Check sheet for the modelled part. Datum: model origin and axes. Units: mm. A direction names the side the tool comes from. Round coordinates to 2 decimals unless told otherwise and drop trailing zeros. Write each loop counter-clockwise with the first axis right and the second up, starting at its lowest first coordinate (ties: lowest second). Pieces come first, ordered by that corner, then holes. Notation, with made-up numbers: (-29, 29) - (7, 29) arc R17 cw to (7, 61) - close; hole circle Ø2 at (21, -39.75). An arc over 180 degrees is marked (long way). Answer as a JSON object with one key per item and string values. Group by question number.
Item 1: Thickness scan on line 1 (Y direction, x = 22.55, z = 0); line 2 (X direction, y = 14.5, z = -7); line 3 (Y direction, x = 6, z = 0). Record the ranges inside material, lowest first.
Item 2: Sectioned sample at A-A on y = 0. Record the boundary of the cut face in (x, z) (3 decimals).
Item 3: Set-up check for faces 1 (the flat face through (22.05, 5, -9)), 2 (the flat face through (12, 0, -4.885)), 3 (the flat face through (24.05, 0, 6)): record each of +Z, -Z, +X, -X, +Y, -Y from which the full face is reachable in a straight line by a thin tool's end or side.
Item 4: Sectioned sample at B-B on x = 16.5. Record the boundary of the cut face in (y, z) (3 decimals).
Item 5: Gauge pin test, flat ends, axial feed: P1, Ø1, axis at x = 18.5, z = 14, coming from the -Y side; P2, Ø3, axis at x = 21, z = -8.5, coming from the +Y side; P3, Ø4, axis at y = 16.5, z = 11.5, coming from the +X side. Record the tip position at first contact, or that the pin passes through.
Item 6: Release check for a two-part mould opening along Y. For faces 4 (the cylindrical face through (2.46, 1.32, 29.97)), 5 (the flat face through (0, 0, -6)), 6 (the flat face through (12.19, 4.21, -2.48)), 7 (the flat face through (12.19, -4.21, 2.48)) record: pulls with the +Y half, pulls with the -Y half, needs draft (parallel to the pull), parting line crosses it, or undercut.
Item 7: Sectioned sample at D-D on y = 26. Record the boundary of the cut face in (x, z).
Item 8: Sectioned sample at C-C on z = 14. Record the boundary of the cut face in (x, y), plus the area to 3 significant figures.
```python
from build123d import *

# Parameters (mm, degrees)
SKETCH2_R           = 30
BOSS_EXTRUDE1_DEPTH = 5
SKETCH3_R           = 15
BOSS_EXTRUDE2_DEPTH = 19.05
CUT_EXTRUDE1_DEPTH  = 24.05
SKETCH5_R           = 2.5
CUT_EXTRUDE2_DEPTH  = 2


with BuildPart() as part:
    # Sketch2 → Boss-Extrude1 (new body)
    with BuildSketch(Plane(origin=(0, 0, 0), x_dir=(0, 0, -1), z_dir=(1, 0, 0))):
        Circle(SKETCH2_R)
    extrude(amount=BOSS_EXTRUDE1_DEPTH)

    # Sketch3 → Boss-Extrude2 (add)
    with BuildSketch(Plane(origin=(5, 0, 0), x_dir=(0, 0, -1), z_dir=(1, 0, 0))):
        with Locations(Location((0, 0, 0), (0, 0, 180))):
            Circle(SKETCH3_R)
    extrude(amount=BOSS_EXTRUDE2_DEPTH)

    # Sketch4 → Cut-Extrude1 (cut)
    with BuildSketch(Plane(origin=(24.05, 0, 0), x_dir=(0, 0, -1), z_dir=(1, 0, 0))):
        Polygon((0, 5.64071213), (-4.885, 2.820356065), (-4.885, -2.820356065), (0, -5.64071213), (4.885, -2.820356065), (4.885, 2.820356065), align=None)
    extrude(amount=-CUT_EXTRUDE1_DEPTH, mode=Mode.SUBTRACT)

    # Sketch5 → Cut-Extrude2 (cut)
    with BuildSketch(Plane(origin=(24.05, 0, 0), x_dir=(0, 0, -1), z_dir=(1, 0, 0))):
        with Locations((8.937690528, 5.160178032)):
            Circle(SKETCH5_R)
        with Locations((-8.937690528, 5.160178032)):
            Circle(SKETCH5_R)
        with Locations((0, -10.320356065)):
            Circle(SKETCH5_R)
    extrude(amount=-CUT_EXTRUDE2_DEPTH, mode=Mode.SUBTRACT)


solid = part.part
```
Completed:
{
 "1": {"line 1": "-15 to -12.82, -7.82 to -5.64, 5.64 to 15", "line 2": "0 to 5", "line 3": "-15 to -5.64, 5.64 to 15"},
 "2": {"outline": "(0, -30) - (5, -30) - (5, -15) - (24.05, -15) - (24.05, -4.885) - (0, -4.885) - close; (0, 4.885) - (24.05, 4.885) - (24.05, 15) - (5, 15) - (5, 30) - (0, 30) - close"},
 "3": {"face 1": "+X", "face 2": "+X, -X", "face 3": "+Z, -Z, +X, +Y, -Y"},
 "4": {"outline": "circle Ø30 at (0, 0); hole (-5.641, 0) - (-2.82, -4.885) - (2.82, -4.885) - (5.641, 0) - (2.82, 4.885) - (-2.82, 4.885) - close"},
 "5": {"P1": "y = -6.54", "P2": "y = 13.27", "P3": "x = 5"},
 "6": {"face 4": "parting line crosses it", "face 5": "needs draft", "face 6": "undercut", "face 7": "undercut"},
 "7": {"outline": "(0, -14.97) - (5, -14.97) - (5, 14.97) - (0, 14.97) - close"},
 "8": {"outline": "(0, -26.53) - (5, -26.53) - (5, -5.39) - (24.05, -5.39) - (24.05, 5.39) - (5, 5.39) - (5, 26.53) - (0, 26.53) - close", "area": "471 mm²"}
}
